The model under review builds one solid part; all positions refer to its coordinate system, in mm. A direction names the side the tool comes from. Coordinates: 2 decimals unless noted, no trailing zeros. Order: outer loops, then holes, each group sorted by start corner. A loop starts at its lowest first (then second) coordinate and runs counter-clockwise, first axis right, second up. Notation, with made-up numbers: (82.25, 48.25) -> (113.25, 48.25) arc R21 ccw to (113.25, 59.25) -> close; hole circle Ø2 at (18.25, 78.5). An arc over 180 degrees is marked (long way). Use one line per item in the form item = value. Start each with the question number.
(1) Insertion check: pin 1 Ø3 at (x, z) = (-2, 5) entering from +Y; pin 2 Ø3 at (x, z) = (29.5, -4.5) entering from -Y; pin 3 Ø1 at (y, z) = (-5.5, 1) entering from +X. Each pin has a flat end and moves straight along its axis. Give the tip position at first contact, or say it passes through.
(2) Mouldability with a two-part tool opening along Z and no side actions: class faces 1 (the flat face through (-8, 0, 4)), 2 (the flat face through (0, 0.1, -5.2)), 3 (the cylindrical face through (-4.44, 1.73, -7.81)) as +Z half, -Z half, draft (parallel to the pull), parting line (faces both ways), or undercut.
(3) Wall thickness on line 1 along X through (y, z) = (4.75, -3.5); line 2 along Y through (x, z) = (30.5, 0.25); line 3 along X through (y, z) = (-2.75, 2.75): over which ranges is each line inside the solid? List them lowest first.
(4) Take a section at A-A (x = 9.5). State the section outline as (y, z) points, then the cut area to 3 significant figures.
(5) For faces 4 (the flat face through (-8, 0, -4)), 5 (the cylindrical face through (22, 5, 0)), 6 (the flat face through (45, 0, 0)), list the 3-axis set-ups (+Z, -Z, +X, -X, +Y, -Y) from which the entire face can be reached by the end or side of a thin tool; tool diameter is ignored.
```python
from build123d import *

# Parameters (mm, degrees)
CUT_EXTRUDE1_DEPTH = 5
CHAMFER1_SIZE      = 1


with BuildPart() as part:
    # Sketch1 → Revolve1 (revolve)
    with BuildSketch(Plane.XY, mode=Mode.PRIVATE) as revolve1_sk:
        Polygon((-10, 0), (-10, 8), (0, 8), (0, 5), (45, 5), (45, 0), align=None)
    revolve(revolve1_sk.sketch.rotate(Axis((45, 0, 0), (-1, 0, 0)), 180), axis=Axis((45, 0, 0), (-1, 0, 0)))

    # Sketch2 → Cut-Revolve1 (revolve, cut)
    with BuildSketch(Plane.XY, mode=Mode.PRIVATE) as cut_revolve1_sk:
        Polygon((-10, 0), (-10, 3.995), (-5, 3.995), (-3.929542976, 0), align=None)
    revolve(cut_revolve1_sk.sketch.rotate(Axis((-3.929542976, 0, 0), (-1, 0, 0)), 180), axis=Axis((-3.929542976, 0, 0), (-1, 0, 0)), mode=Mode.SUBTRACT)

    # Sketch3 → Cut-Extrude1 (cut)
    with BuildSketch(Plane(origin=(-10, 0, 0), x_dir=(0, 0, -1), z_dir=(1, 0, 0))):
        Polygon((0, 4.618802154), (-4, 2.309401077), (-4, -2.309401077), (0, -4.618802154), (4, -2.309401077), (4, 2.309401077), align=None)
    extrude(amount=CUT_EXTRUDE1_DEPTH, mode=Mode.SUBTRACT)

    # Chamfer1
    chamfer1_edges = [part.edges().sort_by_distance(p)[0] for p in [
        (45, 5, 0),
        (-10, 8, 0),
    ]]
    chamfer(chamfer1_edges, length=CHAMFER1_SIZE)


solid = part.part
```
Findings:
q1.pin_1 = 7.19
q1.pin_2 = -4
q1.pin_3 = 0
q2.face_1 = undercut
q2.face_2 = draft
q2.face_3 = parting line
q3.line_1 = -10 to 0
q3.line_2 = -4.99 to 4.99
q3.line_3 = -4.97 to 45
q4.outline = circle Ø10 at (0, 0)
q4.area = 78.5 mm²
q5.face_4 = -X
q5.face_5 = +X
q5.face_6 = +Z, -Z, +X, +Y, -Y
